Autodesk Inventor part; units mm, degrees
ref_plane "YZ Plane" through (0, 0, 0) normal (1, 0, 0) x (0, 1, 0)
ref_plane "XZ Plane" through (0, 0, 0) normal (0, 1, 0) x (-1, 0, 0)
ref_plane "XY Plane" through (0, 0, 0) normal (0, 0, 1) x (1, 0, 0)
sketch "Эскиз1" plane through (0, 0, 0) normal (1, 0, 0) x (0, 1, 0)
  circle A0 centre (25.7199, 46.7921) radius 2.25
  circle A1 centre (25.6987, 6.5017) radius 4.6
  circle A2 centre (7.6987, 6.5017) radius 1.6
  arc A3 (27.6873, 0.2956) -> (32.7199, 5.2955) centre (27.7199, 5.2955) ccw
  circle A4 centre (7.6843, 30.491) radius 14
  arc A5 (14.2267, 42.8683) -> (-1.4853, 19.9118) centre (7.6843, 30.491) ccw
  circle A6 centre (27.6987, 30.491) radius 1.6
  line L0 (7.6843, 30.491) -> (25.6987, 6.5017)
  circle A7 centre (2.6987, 49.5017) radius 1.5
  circle A8 centre (7.6987, 6.5017) radius 3
  line L1 (7.6987, 3.5017) -> (27.6873, 0.2956)
  circle A9 centre (2.6987, 49.5017) radius 3
  line L2 (-3.2958, 40.9198) -> (-5.3755, 35.5348)
  line L3 (-0.0999, 50.5825) -> (-5.3755, 35.5348)
  line L4 (-1.3769, 17.8835) -> (-4.5981, 23.7723)
  line L5 (-4.5981, 23.7723) -> (5.0667, 5.062)
  circle A10 centre (25.7199, 46.7921) radius 4
  line L6 (2.4504, 52.4914) -> (23, 51)
  line L7 (2.4504, 52.4914) -> (26.0094, 50.7816)
  line L8 (32.7199, 5.2955) -> (29.7095, 47.0795)
  point P0 (0, 0)
  point P1 (-2.3427, 0)
  point P2 (7.6843, 30.491)
  point P3 (7.6843, 30.491)
  point P4 (-4.5981, 23.7723)
  point P5 (-3.3371, 41.4181)
  point P6 (-5.3755, 35.5348)
  point P7 (5.0013, 5.1886)
  point P8 (-0.1621, 50.405)
  point P9 (3.376, 52.4242)
  dimension "d132" = 28
  dimension "d9" = 4.5
  dimension "d86" = 9.2
  dimension "d87" = 3.2
  dimension "d92" = 5
  dimension "d145" = 3.2
  dimension "d191" = 30
  dimension "d227" = 3
  dimension "d234" = 6
  dimension "d235" = 6
  dimension "d242" = 8
extrude "Выдавливание1" add sketch "Эскиз1" along normal blind 2.5 contours A8 | A4 L3 A9 L6 L7 A10 L8 A3 L1 A8 L5 | A4 | L6 A9 | A10
equation "\"Радиус_гибки\" = Толщина"
equation "\"Ширина_просечки\" = Толщина"
equation "\"Глубина_просечки\" = 0.5 * Толщина"
equation "\"Размер_просечки\" = 4 * Толщина"
equation "\"Мин_остаток\" = 2 * Толщина"
equation "\"Радиус_перехода\" = Радиус_гибки"
equation "\"Радиус_Якоби\" = Радиус_гибки"
equation "\"Размер_зазора\" = Толщина"
properties part number "drib_lef"
Could you check a few things on this model? Use its own coordinates, in mm. Round coordinates to 2 decimals unless told otherwise and drop trailing zeros. Write each loop counter-clockwise with the first axis right and the second up, starting at its lowest first coordinate (ties: lowest second). Pieces come first, ordered by that corner, then holes. Notation, with made-up numbers: (75.5, -32) - (97.5, -32) arc R28 cw to (97.5, -12) - close; hole circle Ø5 at (-9.75, 60.25). An arc over 180 degrees is marked (long way). Put each result on its own line as item: value. Start each with the question number.
(1) Will these pins go through, and if not, where does the flat tip stop? pin 1 (1.5 mm diameter, centred on x = 1.5, z = 13, fed in from -Y); pin 2 (1 mm diameter, centred on x = 2, z = 43.5, fed in from +Y); pin 3 (1.8 mm diameter, centred on y = 2.7, z = 49.5, fed in from -X).
(2) Thinking about a two-plate mould opening in Y: for faces 1 (the cylindrical face through (1.232, 27.821, 10.583)), 2 (the cylindrical face through (1.23, 28.52, 49.65)), 3 (the cylindrical face through (1.23, 1.27, 52.14)), 4 (the cylindrical face through (1.23, -6.28, 29.48)), which applies, released by +Y, released by -Y, zero draft, split by the parting line, or undercut?
(3) I want a section at C-C, the plane x = 1.4. Please give me the cut outline in (y, z).
(4) I want a section at B-B, the plane y = 2. Please give me the cut outline in (x, z).
(5) I want a section at A-A, the plane y = 24. Please give me the cut outline in (x, z).
(6) I want a section at D-D, the plane z = 40.5. Please give me the cut outline in (x, y).
(7) I need wall thicknesses on probe 1 along Z at (x, y) = (0.3, 2); probe 2 along Z at (x, y) = (1.25, 22); probe 3 along Y at (x, z) = (2, 30.5). Which ranges of each line are inside material? Lowest first, please.
Here are the results:
1. pin 1: stops at y = 0.58
1. pin 2: stops at y = 30
1. pin 3: passes through
2. face 1: undercut
2. face 2: released by +Y
2. face 3: split by the parting line
2. face 4: released by -Y
3. outline: (-5.38, 35.53) arc R14 ccw to (-4.6, 23.77) - (5.07, 5.06) arc R3 ccw to (7.7, 3.5) - (27.69, 0.3) arc R5 ccw to (32.72, 5.3) - (29.71, 47.08) arc R4 ccw to (26.01, 50.78) - (23, 51) - (3.38, 52.42) arc R3 ccw to (-0.1, 50.58) - close; hole circle Ø3 at (2.7, 49.5); hole circle Ø3.2 at (7.7, 6.5); hole circle Ø9.2 at (25.7, 6.5); hole circle Ø4.5 at (25.72, 46.79); hole circle Ø3.2 at (27.7, 30.49)
4. outline: (0, 11) - (2.5, 11) - (2.5, 48.17) - (0, 48.17) - close; (0, 50.83) - (2.5, 50.83) - (2.5, 52.42) - (0, 52.42) - close
5. outline: (0, 0.89) - (2.5, 0.89) - (2.5, 2.23) - (0, 2.23) - close; (0, 10.78) - (2.5, 10.78) - (2.5, 45.34) - (0, 45.34) - close; (0, 48.24) - (2.5, 48.24) - (2.5, 50.93) - (0, 50.93) - close
6. outline: (0, -3.63) - (2.5, -3.63) - (2.5, 30.18) - (0, 30.18) - close
7. probe 1: z = 11 to 48.17, 50.83 to 52.42
7. probe 2: z = 1.21 to 3.77, 9.24 to 51.07
7. probe 3: y = -6.32 to 26.1, 29.3 to 30.9
